from build123d import *

# Parameters (mm, degrees)
F0_W      = 50
F0_H      = 40
F1_DEPTH  = 30
F2_W      = 10
F2_H      = 10
F3_DEPTH  = 50
F3_FACE_W = 10
F3_FACE_H = 10
F4_DEPTH  = 100


with BuildPart() as f1:
    # F0 (on Front) → F1 (new body)
    with BuildSketch(Plane.XZ):
        with Locations((25, 20)):
            Rectangle(F0_W, F0_H)
    extrude(amount=F1_DEPTH)

    # F2 (on face) → F3 (join)
    with BuildSketch(Plane.YZ.offset(50)):
        with Locations((-15, 35)):
            Rectangle(F2_W, F2_H)
    extrude(amount=F3_DEPTH)

    # F3_face (on face) → F4 (cut)
    with BuildSketch(Plane(origin=(100, -15, 35), x_dir=(0, 1, 0), z_dir=(1, 0, 0))):
        Rectangle(F3_FACE_W, F3_FACE_H)
    extrude(amount=-F4_DEPTH, mode=Mode.SUBTRACT)


solid = f1.part
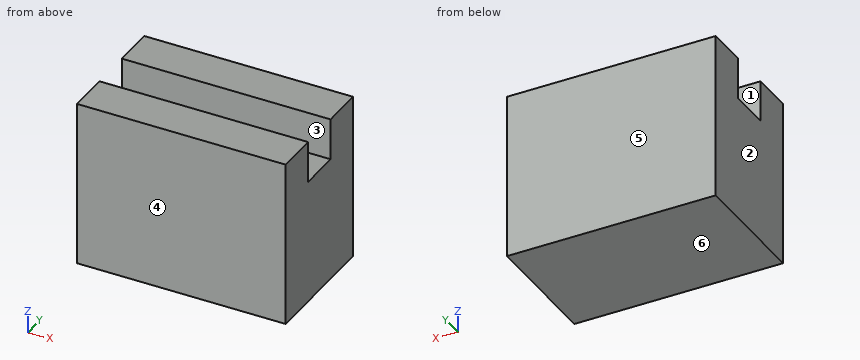
Geometry check sheet. Reference: the model listing, model coordinates, mm. Face numbers are marked on the shaded views. A direction names the side the tool comes from. Coordinates: 2 decimals unless noted, no trailing zeros. Order: outer loops, then holes, each group sorted by start corner. A loop starts at its lowest first (then second) coordinate and runs counter-clockwise, first axis right, second up. Notation, with made-up numbers: (78, 69) - (89, 69) arc R20 cw to (89, 97) - close; hole circle Ø5 at (43, 88.5). An arc over 180 degrees is marked (long way). Answer in a Markdown table with one row per item. Add a question column.
1) Release check for a two-part mould opening along Y. For the marked faces 3, 4, 5 and 6 record: +Y half, -Y half, draft (parallel to the pull), parting line (faces both ways), or undercut.
2) Gauge pin test, flat end, axial feed: P1, Ø3, axis at y = -12, z = 10, coming from the -X side. Record the tip position at first contact, or that the pin passes through.
3) Material ranges on line 1 along Y through (x, z) = (20.5, 37); line 2 along Z through (x, y) = (48, -12), recorded low to high. Write a range as [from, to].
4) Set-up check for the marked faces 1 and 2: record each of +Z, -Z, +X, -X, +Y, -Y from which the full face is reachable in a straight line by a thin tool's end or side.
5) Cross-section at C-C, the plane y = -13.5. Record the cut outline in (x, z), then the cut area to 3 significant figures.
6) Cross-section at A-A, the plane z = 35.5. Record the cut outline in (x, y), then the cut area to 3 significant figures.
7) Cross-section at B-B, the plane x = 23.5. Record the cut outline in (y, z), then the cut area to 3 significant figures.
Check result:
| question | item | result |
|---|---|---|
| 1 | face 3 | undercut |
| 1 | face 4 | -Y half |
| 1 | face 5 | +Y half |
| 1 | face 6 | draft |
| 2 | P1 | stops at x = 0 |
| 3 | line 1 | y = [-30, -20], [-10, 0] |
| 3 | line 2 | z = [0, 30] |
| 4 | face 1 | +Z, +X, -X |
| 4 | face 2 | +Z, -Z, -X, +Y, -Y |
| 5 | outline | (0, 0) - (50, 0) - (50, 30) - (0, 30) - close |
| 5 | area | 1,500 mm² |
| 6 | outline | (0, -30) - (50, -30) - (50, -20) - (0, -20) - close; (0, -10) - (50, -10) - (50, 0) - (0, 0) - close |
| 6 | area | 1,000 mm² |
| 7 | outline | (-30, 0) - (0, 0) - (0, 40) - (-10, 40) - (-10, 30) - (-20, 30) - (-20, 40) - (-30, 40) - close |
| 7 | area | 1,100 mm² |
